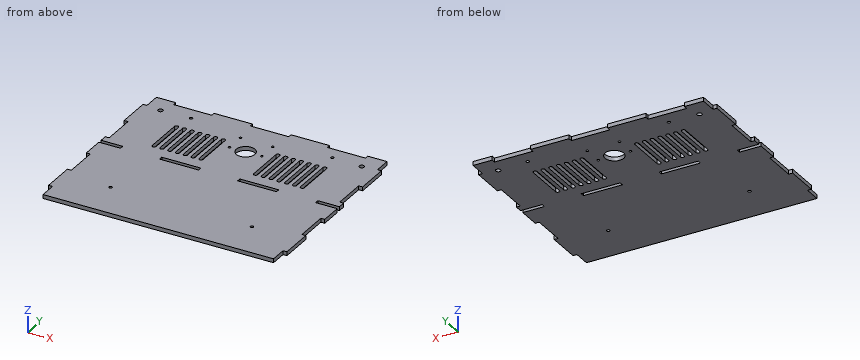
```python
from build123d import *

# Parameters (mm, degrees)
SKETCH1_W                      = 150.114
SKETCH1_H                      = 129.54
BOSS_EXTRUDE1_DEPTH            = 2.54
SKETCH4_W                      = 25.019
SKETCH4_H                      = 2.54
CUT_EXTRUDE1_DEPTH             = 100.172363837
LPATTERN1_COUNT                = 3
LPATTERN1_PITCH                = 50.038
SKETCH5_W                      = 2.54
SKETCH5_H                      = 21.59
BOSS_EXTRUDE3_DEPTH            = 2.54
LPATTERN2_COUNT                = 3
LPATTERN2_PITCH                = 43.18
LPATTERN2_COUNT_DIR2           = 2
LPATTERN2_PITCH_DIR2           = 152.654
TAP_DRILL_FOR_M2_5X0_45_TAP1_D = 2.05
M3_CLEARANCE_HOLE1_D           = 3.2
M3_CLEARANCE_HOLE1_DEPTH       = 9.398
M3_CLEARANCE_HOLE1_TIP         = 0.96137699
SKETCH10_R                     = 6.096
CUT_EXTRUDE2_DEPTH             = 102.108352321
TAP_DRILL_FOR_M2X0_4_TAP1_D    = 1.6
SKETCH13_W                     = 25.4
SKETCH13_H                     = 2.54
CUT_EXTRUDE3_DEPTH             = 102.108352321
CUT_EXTRUDE4_DEPTH             = 102.108352321
LPATTERN3_COUNT                = 7
LPATTERN3_PITCH                = 5.08
LPATTERN3_COUNT_DIR2           = 14
LPATTERN3_PITCH_DIR2           = 5.08


with BuildPart() as part:
    # Sketch1 → Boss-Extrude1 (new body)
    with BuildSketch(Plane.XY):
        Rectangle(SKETCH1_W, SKETCH1_H)
    extrude(amount=BOSS_EXTRUDE1_DEPTH)

    # Sketch4 → Cut-Extrude1 (cut, through all)
    with BuildSketch(Plane.XY.offset(2.54)):
        with Locations((-50.038, 63.5)):
            Rectangle(SKETCH4_W, SKETCH4_H)
    cut_extrude1 = extrude(amount=-CUT_EXTRUDE1_DEPTH, mode=Mode.SUBTRACT)

    # LPattern1: Cut-Extrude1 ×3
    with Locations(*[(i * LPATTERN1_PITCH, 0, 0) for i in range(1, LPATTERN1_COUNT)]):
        add(cut_extrude1, mode=Mode.SUBTRACT)

    # Sketch5 → Boss-Extrude3 (add)
    with BuildSketch(Plane.XY.offset(2.54)):
        with Locations((-76.327, 43.18)):
            Rectangle(SKETCH5_W, SKETCH5_H)
    boss_extrude3 = extrude(amount=-BOSS_EXTRUDE3_DEPTH)

    # LPattern2: Boss-Extrude3 3 × 2
    with Locations(*[(j * LPATTERN2_PITCH_DIR2, -i * LPATTERN2_PITCH, 0) for i in range(LPATTERN2_COUNT) for j in range(LPATTERN2_COUNT_DIR2) if (i, j) != (0, 0)]):
        add(boss_extrude3)

    # Tap Drill for M2.5x0.45 Tap1 (through all)
    with Locations(Plane.XY.offset(2.54)):
        with Locations((46, 53.413478245), (-45.9999938, 53.413478245), (-45.9999938, -38.586515555), (46, -38.586515555)):
            Hole(TAP_DRILL_FOR_M2_5X0_45_TAP1_D / 2)

    # M3 Clearance Hole1
    with Locations(Plane.XY.offset(2.54)):
        with Locations((-65.532, 52.705), (65.532, 52.705)):
            Hole(M3_CLEARANCE_HOLE1_D / 2, depth=M3_CLEARANCE_HOLE1_DEPTH)
            with Locations((0, 0, -(M3_CLEARANCE_HOLE1_DEPTH + M3_CLEARANCE_HOLE1_TIP / 2))):  # 118° drill point
                Cone(0, M3_CLEARANCE_HOLE1_D / 2, M3_CLEARANCE_HOLE1_TIP, mode=Mode.SUBTRACT)

    # Sketch10 → Cut-Extrude2 (cut, through all)
    with BuildSketch(Plane(origin=(0, 0, 0), x_dir=(-1, 0, 0), z_dir=(0, 0, -1))):
        with Locations((0, 34.98)):
            Circle(SKETCH10_R)
    extrude(amount=-CUT_EXTRUDE2_DEPTH, mode=Mode.SUBTRACT)

    # Tap Drill for M2x0.4 Tap1 (through all)
    with Locations(Plane(origin=(0, 0, 0), x_dir=(-1, 0, 0), z_dir=(0, 0, -1))):
        with Locations((-10.5, 47.53), (-10.5, 35.03), (10.5, 47.53), (10.5, 35.03)):
            Hole(TAP_DRILL_FOR_M2X0_4_TAP1_D / 2)

    # Sketch13 → Cut-Extrude3 (cut, through all)
    with BuildSketch(Plane.XY.offset(2.54)):
        with Locations((-25.4, 4.7625)):
            Rectangle(SKETCH13_W, SKETCH13_H)
        with Locations((-76.2, 4.7625)):
            Rectangle(SKETCH13_W, SKETCH13_H)
    cut_extrude3 = extrude(amount=-CUT_EXTRUDE3_DEPTH, mode=Mode.SUBTRACT)

    # Mirror1: Cut-Extrude3 across plane
    add(cut_extrude3.mirror(Plane(origin=(0, 0, 0), x_dir=(0, 0, 1), z_dir=(1, 0, 0))), mode=Mode.SUBTRACT)

    # Sketch14 → Cut-Extrude4 (cut, through all)
    with BuildSketch(Plane.XY.offset(2.54)):
        with BuildLine():
            Line((-16.51, 40.64), (-16.51, 15.24))
            ThreePointArc((-16.51, 15.24), (-17.78, 13.97), (-19.05, 15.24))
            Line((-19.05, 15.24), (-19.05, 40.64))
            ThreePointArc((-19.05, 40.64), (-17.78, 41.91), (-16.51, 40.64))
        make_face()
    cut_extrude4 = extrude(amount=-CUT_EXTRUDE4_DEPTH, mode=Mode.SUBTRACT)

    # LPattern3: Cut-Extrude4 7 × 14, 42 skipped
    with Locations(*[Vector(-1, 0, 0) * (i * LPATTERN3_PITCH) + Vector(1, 0, 0) * (j * LPATTERN3_PITCH_DIR2) for i in range(LPATTERN3_COUNT) for j in range(LPATTERN3_COUNT_DIR2) if (i, j) not in ((0, 0), (0, 1), (0, 2), (0, 3), (0, 4), (0, 5), (0, 6), (1, 2), (1, 3), (1, 4), (1, 5), (1, 6), (1, 7), (2, 3), (2, 4), (2, 5), (2, 6), (2, 7), (2, 8), (3, 4), (3, 5), (3, 6), (3, 7), (3, 8), (3, 9), (4, 5), (4, 6), (4, 7), (4, 8), (4, 9), (4, 10), (5, 6), (5, 7), (5, 8), (5, 9), (5, 10), (5, 11), (6, 7), (6, 8), (6, 9), (6, 10), (6, 11), (6, 12))]):
        add(cut_extrude4, mode=Mode.SUBTRACT)


solid = part.part
```
Can you work these out from the model? Positions are in its coordinate system, mm. Give positions to 0.01 mm unless a question says otherwise; leave off trailing zeros. Write each loop counter-clockwise with the first axis right and the second up, starting at its lowest first coordinate (ties: lowest second). Pieces come first, ordered by that corner, then holes. Notation, with made-up numbers: (-13, -22) - (-2, -22) arc R22 cw to (-2, 11) - close; hole circle Ø4 at (53, -40). An arc over 180 degrees is marked (long way). Write item = value, one per line. Start each with the question number.
1. Imagine slicing it at A-A (x = 0). Please give me the cut outline in (y, z), and give its area (3 significant figures).
2. Imagine slicing it at C-C (y = -28). Please give me the cut outline in (x, z).
3. For pin 1 (1.3 mm diameter, centred on y = -17, z = 2, fed in from -X); pin 2 (0.8 mm diameter, centred on y = 5.5, z = 1, fed in from +X); pin 3 (0.8 mm diameter, centred on x = 76, z = 1, fed in from +Y) (3 decimals), each with a flat end and sliding along its axis, tell me the tip position at first contact or that it passes through.
4. Imagine slicing it at D-D (z = 2.1). Count the separate pieces of the cut face and the enclosed holes in it, and give its area (3 significant figures).
5. Please list where these lines run through material, in increasing order: line 1 (Y direction, x = 46, z = 0.7); line 2 (Y direction, x = -10.5, z = 1.8); line 3 (X direction, y = 52, z = 1).
6. Imagine slicing it at B-B (x = -55.5). Please give me the cut outline in (y, z).
Worked answers:
q1.outline = (-64.77, 0) - (28.88, 0) - (28.88, 2.54) - (-64.77, 2.54) - close; (41.08, 0) - (62.23, 0) - (62.23, 2.54) - (41.08, 2.54) - close
q1.area = 292 mm2
q2.outline = (-75.06, 0) - (75.06, 0) - (75.06, 2.54) - (-75.06, 2.54) - close
q3.pin_1 = -75.06
q3.pin_2 = 63.5
q3.pin_3 = 53.975
q4.separate_pieces = 1
q4.enclosed_holes = 27
q4.area = 18,300 mm2
q5.line_1 = -64.77 to -39.61, -37.56 to 52.39, 54.44 to 62.23
q5.line_2 = -64.77 to 34.23, 35.83 to 46.73, 48.33 to 62.23
q5.line_3 = -77.6 to -66.97, -64.1 to 64.1, 66.97 to 77.6
q6.outline = (-64.77, 0) - (62.23, 0) - (62.23, 2.54) - (-64.77, 2.54) - close
